from build123d import *

# Parameters (mm, degrees)
F1_DEPTH = 25
F2_DEPTH = 5
F0_W     = 10
F0_H     = 7.5000003082
F3_DEPTH = 10


with BuildPart() as f1:
    # F0 (on Front) → F1 (new body, symmetric)
    with BuildSketch(Plane.XZ):
        Polygon((-16.25, 3.75), (-16.25, -3.75), (16.25, -3.75), (16.25, 3.75), (8.7499996918, 3.75), align=None)
    extrude(amount=F1_DEPTH, both=True)

    # F0 (on Front) → F2 (join, symmetric)
    with BuildSketch(Plane.XZ):
        with BuildLine():
            add(Edge.make_bspline(
                [(21.8955707276, 24.3667089847), (-3.4341610337, 23.7179701403), (-15.9380340583, 11.8111578561), (-16.25, 3.75)],
                knots=[0.3450535136, 0.3450535136, 0.3450535136, 0.3450535136, 43.8994238312, 43.8994238312, 43.8994238312, 43.8994238312], degree=3))
            Line((-16.25, 3.75), (8.7499996918, 3.75))
            Line((8.7499996918, 3.75), (8.7499996918, 10.63))
            ThreePointArc((8.7499996918, 10.63), (12.5658817413, 20.1366188993), (21.8955707276, 24.3667089847))
        make_face()
    extrude(amount=F2_DEPTH, both=True)

    # F0 (on Front) → F3 (join, symmetric)
    with BuildSketch(Plane.XZ):
        with BuildLine():
            Line((8.7499996918, 3.75), (16.25, 3.75))
            Line((16.25, 3.75), (16.25, 10.63))
            ThreePointArc((16.25, 10.63), (18.0805826176, 15.0494173824), (22.5, 16.88))
            Line((22.5, 16.88), (23.75, 16.88))
            Line((23.75, 16.88), (23.75, 24.3800003082))
            Line((23.75, 24.3800003082), (22.5, 24.3800003082))
            add(Edge.make_bspline(
                [(22.5, 24.3800003082), (22.2977183657, 24.3762814735), (22.0962420467, 24.371848529), (21.8955707276, 24.3667089847)],
                knots=[0, 0, 0, 0, 0.3450535136, 0.3450535136, 0.3450535136, 0.3450535136], degree=3))
            ThreePointArc((21.8955707276, 24.3667089847), (12.5658817413, 20.1366188993), (8.7499996918, 10.63))
            Line((8.7499996918, 10.63), (8.7499996918, 3.75))
        make_face()
        with Locations((28.75, 20.6300001541)):
            Rectangle(F0_W, F0_H)
    extrude(amount=F3_DEPTH, both=True)

    # F0 (on Front) → F4 (revolve)
    with BuildSketch(Plane.XZ):
        Polygon((33.75, 26.25), (33.75, 24.3800003082), (33.75, 16.88), (33.75, 15), (43.75, 15), (43.75, 26.25), align=None)
    revolve(axis=Axis((33.75, 0, 20.625), (0, 0, -1)))


solid = f1.part
Can you work these out from the model? Positions are in its coordinate system, mm. A direction names the side the tool comes from. Coordinates: 2 decimals unless noted, no trailing zeros. Write each loop counter-clockwise with the first axis right and the second up, starting at its lowest first coordinate (ties: lowest second). Pieces come first, ordered by that corner, then holes. Notation, with made-up numbers: (-3, 87) - (56, 87) arc R20 ccw to (56, 115) - close; hole circle Ø9 at (56.25, 70.5). An arc over 180 degrees is marked (long way). Return JSON: item names as keys, results as strings. Group by question number.
Item 1: I'm going to push flat-ended pins straight in: pin 1 Ø2.5 at (y, z) = (-8, 6) entering from -X; pin 2 Ø10 at (y, z) = (12.5, 8.5) entering from +X; pin 3 Ø5.5 at (x, y) = (27, -3) entering from -Z; pin 4 Ø6 at (x, z) = (-2.5, 6.5) entering from -Y. Where does each tip first touch, or does it pass through?
Item 2: Please list where these lines run through material, in increasing order: probe 1 along Y at (x, z) = (-9, 4.5); probe 2 along X at (y, z) = (10, -2); probe 3 along Y at (x, z) = (13, 4.75).
Item 3: If we section it at A-A (z = 0.25): Write out the boundary of the cut face in (x, y), then the cut area to 4 significant figures.
Item 4: Which directions (+Z, -Z, +X, -X, +Y, -Y) give clear straight access to the entire face, cutting with the end or side of a thin tool? Please do faces 1 (the face through (16.25, 0, 2)), 2 (the face through (18, -10, 17)), 3 (the face through (12.668, -7.535, 20.242)).
Item 5: If we section it at B-B (y = 21): Write out the boundary of the cut face in (x, z), then the cut area to 3 significant figures.
Return value:
{
 "1": {"pin 1": "stops at x = 8.75", "pin 2": "stops at x = 16.65", "pin 3": "stops at z = 15", "pin 4": "stops at y = -25"},
 "2": {"probe 1": "y = -5 to 5", "probe 2": "x = -16.25 to 16.25", "probe 3": "y = -10 to 10"},
 "3": {"outline": "(-16.25, -25) - (16.25, -25) - (16.25, 25) - (-16.25, 25) - close", "area": "1,625 mm^2"},
 "4": {"face 1": "-Z, +X, +Y, -Y", "face 2": "+Z, +X, -X, -Y", "face 3": "+Z, -X, -Y"},
 "5": {"outline": "(-16.25, -3.75) - (16.25, -3.75) - (16.25, 3.75) - (-16.25, 3.75) - close", "area": "244 mm^2"}
}
